Part model, mm, in its own coordinate system. Face numbers are marked on the shaded views. A direction names the side the tool comes from. Give positions to 0.01 mm unless a question says otherwise; leave off trailing zeros. Order: outer loops, then holes, each group sorted by start corner. A loop starts at its lowest first (then second) coordinate and runs counter-clockwise, first axis right, second up. Notation, with made-up numbers: (2.25, 41) -> (38.25, 41) arc R4 ccw to (38.25, 45) -> close; hole circle Ø10 at (40, 75). An arc over 180 degrees is marked (long way). Write item = value, one per line. Start each with the question number.
Item 1: Band-saw the part on D-D on y = 5.5. Write the cut outline in (x, z).
Item 2: Drill centre lines: line 1 along Y through (x, z) = (-0.65, 0); line 2 along Y through (x, z) = (2.5, 1); line 3 along Y through (x, z) = (-1.75, 0.5). Where is each one in solid material? Low to high.
Item 3: Pull direction Z, two halves, no side cores. Call the marked faces 1, 2 and 3: +Z half, -Z half, draft (parallel to the pull), parting line (faces both ways), or undercut.
Item 4: Band-saw the part on A-A on z = 0. Write the cut outline in (x, y), plus the area to 3 significant figures.
Item 5: Band-saw the part on B-B on y = 9.05. Write the cut outline in (x, z), plus the area to 4 significant figures.
Item 6: Tool access for the marked faces 4, 5 and 6: list every direction of +Z, -Z, +X, -X, +Y, -Y with a clear straight run to the whole face (end or side of a thin tool).
Item 7: Band-saw the part on C-C on x = 1.75. Count the separate pieces of the cut face and the enclosed holes in it, plus the area to 3 significant figures.
Item 8: Flat gauge pin, fed straight in: P1, Ø1.2, axis at y = -8, z = 0, coming from the -X side. Where does the tip first touch, or does it go through?
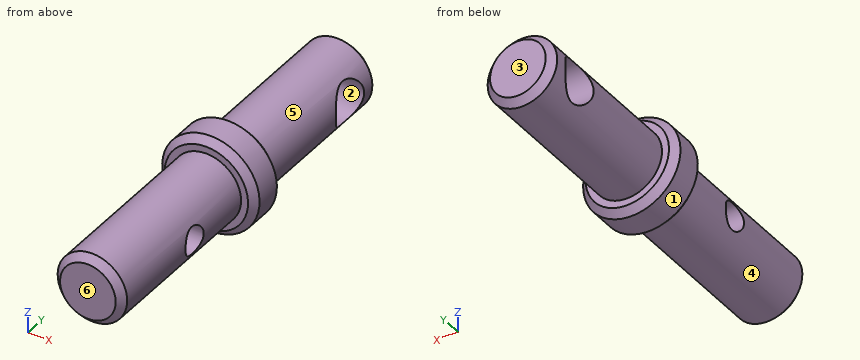
```python
from build123d import *

# Parameters (mm, degrees)
F2_SIZE  = 0.5
F3_R     = 1
F3_R_2   = 1.55
F4_DEPTH = 12.5


with BuildPart() as f1:
    # F0 (on Right) → F1 (revolve)
    with BuildSketch(Plane.YZ):
        Polygon((-15.9, 2.5), (-15.9, 0), (10, 0), (12, 0), (12, 2.5), (4, 2.5), (0, 2.5), (0, 3.5), (-2.9, 3.5), (-2.9, 2.5), align=None)
    revolve(axis=Axis((0, -0.324999528, 0), (0, 1, 0)))

    # F2
    f2_edges = [f1.edges().sort_by_distance(p)[0] for p in [
        (0, -15.9, -2.5),
        (0, 0, -3.5),
        (0, -2.9, -3.5),
        (0, -1.45, 3.5),
        (0, 12, -2.5),
    ]]
    chamfer(f2_edges, length=F2_SIZE)

    # F3 (on Right) → F4 (cut, symmetric)
    with BuildSketch(Plane.YZ):
        with Locations((-8, 0)):
            Circle(F3_R)
        with Locations((9.05, 0)):
            Circle(F3_R_2)
    extrude(amount=F4_DEPTH, both=True, mode=Mode.SUBTRACT)


solid = f1.part
```
Values found:
q1.outline = circle Ø5 at (0, 0)
q2.line_1 = -15.9 to -9, -7 to 7.5, 10.6 to 12
q2.line_2 = -2.9 to 0
q2.line_3 = -15.9 to -8.87, -7.13 to 7.58, 10.52 to 12
q3.face_1 = parting line
q3.face_2 = undercut
q3.face_3 = draft
q4.outline = (-3.5, -2.4) -> (-3, -2.9) -> (-2.5, -2.9) -> (-2.5, -7) -> (2.5, -7) -> (2.5, -2.9) -> (3, -2.9) -> (3.5, -2.4) -> (3.5, -0.5) -> (3, 0) -> (2.5, 0) -> (2.5, 7.5) -> (-2.5, 7.5) -> (-2.5, 0) -> (-3, 0) -> (-3.5, -0.5) -> close; (-2.5, -15.4) -> (-2, -15.9) -> (2, -15.9) -> (2.5, -15.4) -> (2.5, -9) -> (-2.5, -9) -> close; (-2.5, 10.6) -> (2.5, 10.6) -> (2.5, 11.5) -> (2, 12) -> (-2, 12) -> (-2.5, 11.5) -> close
q4.area = 119 mm^2
q5.outline = (-1.96, -1.55) arc R2.5 ccw to (1.96, -1.55) -> close; (-1.96, 1.55) -> (1.96, 1.55) arc R2.5 ccw to start
q5.area = 5.195 mm^2
q6.face_4 = -Y
q6.face_5 = +Y
q6.face_6 = +Z, -Z, +X, -X, -Y
q7.separate_pieces = 1
q7.enclosed_holes = 2
q7.area = 94.8 mm^2
q8.P1 = through
